Could you check a few things on this drawing? It's one solid part, dimensions in mm from its lowest x, y, z. Round coordinates to 2 decimals unless told otherwise and drop trailing zeros. Loops run counter-clockwise (first coordinate to the right, second up) from the corner with the lowest first, then second, coordinate; pieces in that order, holes last. Notation, with made-up numbers: (39, -13) -> (65, -13) arc R7 ccw to (65, -2) -> close; hole circle Ø5 at (24, 4.5). An arc over 180 degrees is marked (long way). Put each result on its own line as item: value. Start each with the question number.
1. Imagine slicing it at C-C, the plane z = 25. Count the separate pieces of the cut face and the enclosed holes in it, and give its area (3 significant figures).
2. Imagine slicing it at A-A, the plane x = 192. Please give me the cut outline in (y, z), and give its area (3 significant figures).
3. Imagine slicing it at B-B, the plane y = 158. Please give me the cut outline in (x, z).
4. If we mould it in two halves opening along Y, with no side actions, what happens to the marked faces 1 and 2? For each: pulls with the +Y half, pulls with the -Y half, needs draft (parallel to the pull), parting line crosses it, or undercut.
5. I'm going to push a flat-ended pin straight in: P1, Ø12, axis at x = 69.5, y = 21, coming from the +Z side. Where does the tip first touch, or does it pass through?
6. I need wall thicknesses on line 1 (X direction, y = 160, z = 24); line 2 (Y direction, x = 37.5, z = 11.5); line 3 (Z direction, x = 154, y = 21.5). Which ranges of each line are inside material? Lowest first, please. Write a range as [from, to].
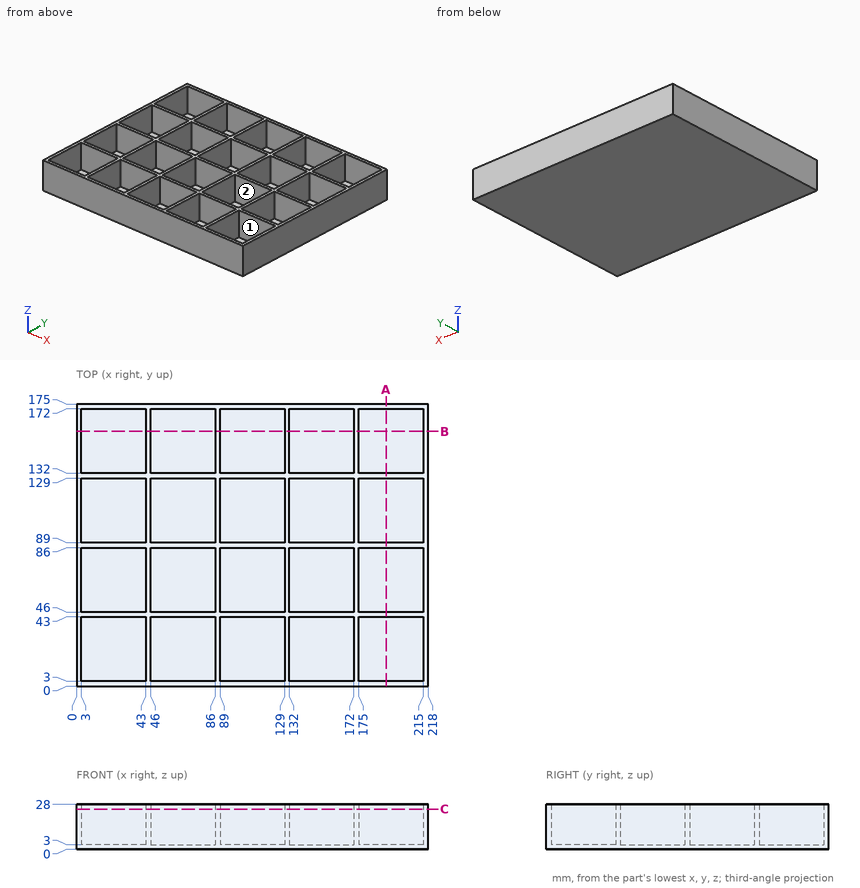
Entries:
1. separate pieces: 1
1. enclosed holes: 20
1. area: 6,150 mm^2
2. outline: (0, 0) -> (175, 0) -> (175, 28) -> (172, 28) -> (172, 3) -> (132, 3) -> (132, 28) -> (129, 28) -> (129, 3) -> (89, 3) -> (89, 28) -> (86, 28) -> (86, 3) -> (46, 3) -> (46, 28) -> (43, 28) -> (43, 3) -> (3, 3) -> (3, 28) -> (0, 28) -> close
2. area: 900 mm^2
3. outline: (0, 0) -> (218, 0) -> (218, 28) -> (215, 28) -> (215, 3) -> (175, 3) -> (175, 28) -> (172, 28) -> (172, 3) -> (132, 3) -> (132, 28) -> (129, 28) -> (129, 3) -> (89, 3) -> (89, 28) -> (86, 28) -> (86, 3) -> (46, 3) -> (46, 28) -> (43, 28) -> (43, 3) -> (3, 3) -> (3, 28) -> (0, 28) -> close
4. face 1: undercut
4. face 2: undercut
5. P1: z = 3
6. line 1: [0, 3], [43, 46], [86, 89], [129, 132], [172, 175], [215, 218]
6. line 2: [0, 3], [43, 46], [86, 89], [129, 132], [172, 175]
6. line 3: [0, 3]
